The listing builds one solid part. Answer for the finished solid, in the listing's coordinates (mm). A direction names the side the tool comes from. Round coordinates to 2 decimals unless told otherwise and drop trailing zeros. Write each loop counter-clockwise with the first axis right and the second up, starting at its lowest first coordinate (ties: lowest second). Pieces come first, ordered by that corner, then holes.
(1) A cutting plane is placed at A-A, the plane y = -1. Give the vertices of the cut face in (x, z).
(2) A cutting plane is placed at B-B, the plane x = 16. Give the vertices of the cut face in (y, z), and give its area (3 significant figures).
(3) Find the intervals of material crossed by probe 1 along Z at (x, y) = (0, 12); probe 2 along Z at (x, y) = (6, -12); probe 3 along Z at (x, y) = (-20.5, -36), in increasing order.
(4) For faces 4 (the face through (-2.219, -15.021, 12.743)), 5 (the face through (20, -39.5, 10)), 6 (the face through (-16.8, -21, 11)), 7 (the face through (-12.897, -3.491, 19.947)), determine the directions among +Z, -Z, +X, -X, +Y, -Y from which every point of the face is accessible in a straight line to the end or side of a thin tool.
(5) A cutting plane is placed at D-D, the plane y = 5.5. Give the vertices of the cut face in (x, z).
(6) The mould has two halves that part along Y. Classify faces 1 (the face through (2.053, -3.491, 34.639)), 2 (the face through (1.3, -13.5, 12.9)), 3 (the face through (-22, -12, 22)): +Y half, -Y half, draft (parallel to the pull), parting line (faces both ways), or undercut.
(7) A cutting plane is placed at C-C, the plane y = -24.5. Give the number of separate pieces and of enclosed holes in the cut face, and give its area (3 significant figures).
from build123d import *

# Parameters (mm, degrees)
F0_R      = 2.05
F1_DEPTH  = 44
F2_R      = 4
F3_DEPTH  = 12.001
F4_DEPTH  = 6.8
F6_DEPTH  = 33.001
F7_R      = 2.05
F8_DEPTH  = 44.001
F9_DEPTH  = 8
F10_R     = 2
F11_DEPTH = 44.001
F12_DEPTH = 3.4
F13_R     = 3.6
F14_DEPTH = 4.2
F16_DEPTH = 44.001
F18_DEPTH = 44.001
F19_R     = 1.55
F20_DEPTH = 33.001
F21_DEPTH = 3


with BuildPart() as f1:
    # F0 (on Top) → F1 (new body)
    with BuildSketch(Plane.XY):
        Polygon((16.5, 16.5), (-16.5, 16.5), (-22, 16.5), (-22, -32.5), (-10, -32.5), (-10, -16.5), (8, -16.5), (8, -32.5), (22, -32.5), (22, 16.5), align=None)
        with Locations((-12, -12)):
            Circle(F0_R, mode=Mode.SUBTRACT)
        with Locations((12, -12)):
            Circle(F0_R, mode=Mode.SUBTRACT)
        with Locations((-12, 12)):
            Circle(F0_R, mode=Mode.SUBTRACT)
        with Locations((12, 12)):
            Circle(F0_R, mode=Mode.SUBTRACT)
    extrude(amount=F1_DEPTH)

    # F2 (on face) → F3 (cut, through all)
    with BuildSketch(Plane.YZ.offset(-10)):
        with Locations((-24.5, 36.4)):
            Circle(F2_R)
        with Locations((-24.5, 22)):
            Circle(F2_R)
        with Locations((-24.5, 7.6)):
            Circle(F2_R)
    extrude(amount=-F3_DEPTH, mode=Mode.SUBTRACT)

    # F2 (on face) → F4 (cut)
    with BuildSketch(Plane.YZ.offset(-10)):
        Polygon((-16.9944465005, 36.4), (-20.7472232503, 42.9), (-28.2527767497, 42.9), (-32.0055534995, 36.4), (-28.2527767497, 29.9), (-20.7472232503, 29.9), align=None)
        with Locations((-24.5, 36.4)):
            Circle(F2_R, mode=Mode.SUBTRACT)
        Polygon((-16.9944465005, 22), (-20.7472232503, 28.5), (-28.2527767497, 28.5), (-32.0055534995, 22), (-28.2527767497, 15.5), (-20.7472232503, 15.5), align=None)
        with Locations((-24.5, 22)):
            Circle(F2_R, mode=Mode.SUBTRACT)
        Polygon((-28.2527767497, 14.1), (-32.0055534995, 7.6), (-28.2527767497, 1.1), (-20.7472232503, 1.1), (-16.9944465005, 7.6), (-20.7472232503, 14.1), align=None)
        with Locations((-24.5, 7.6)):
            Circle(F2_R, mode=Mode.SUBTRACT)
    extrude(amount=-F4_DEPTH, mode=Mode.SUBTRACT)

    # F5 (on face) → F6 (cut, through all)
    with BuildSketch(Plane.XZ.offset(16.5)):
        Polygon((2.0710678119, 27), (-2.0710678119, 27), (-5, 24.0710678119), (-5, 19.9289321881), (-2.0710678119, 17), (2.0710678119, 17), (5, 19.9289321881), (5, 24.0710678119), align=None)
    extrude(amount=-F6_DEPTH, mode=Mode.SUBTRACT)

    # F7 (on face) → F8 (cut, through all)
    with BuildSketch(Plane(origin=(-22, 0, 0), x_dir=(0, -1, 0), z_dir=(-1, 0, 0))):
        with Locations((-12, 34)):
            Circle(F7_R)
        with Locations((12, 34)):
            Circle(F7_R)
        with Locations((12, 10)):
            Circle(F7_R)
        with Locations((-12, 10)):
            Circle(F7_R)
    extrude(amount=-F8_DEPTH, mode=Mode.SUBTRACT)

    # F9 (add): faces of the model
    f9_faces = [f1.faces().sort_by_distance(p)[0] for p in [
        (15, -32.5, 22),
        (-16, -32.5, 22),
    ]]
    extrude(f9_faces, amount=F9_DEPTH)

    # F10 (on face) → F11 (cut, through all)
    with BuildSketch(Plane.YZ.offset(22)):
        with Locations((-36, 10)):
            Circle(F10_R)
        with Locations((-36, 34)):
            Circle(F10_R)
    extrude(amount=-F11_DEPTH, mode=Mode.SUBTRACT)

    # F10 (on face) → F12 (cut)
    with BuildSketch(Plane.YZ.offset(22)):
        Polygon((-32.5, 7.9792740578), (-32.5, 12.0207259422), (-36, 14.0414518843), (-39.5, 12.0207259422), (-39.5, 7.9792740578), (-36, 5.9585481157), align=None)
        with Locations((-36, 10)):
            Circle(F10_R, mode=Mode.SUBTRACT)
        Polygon((-32.5, 31.9792740578), (-32.5, 36.0207259422), (-36, 38.0414518843), (-39.5, 36.0207259422), (-39.5, 31.9792740578), (-36, 29.9585481157), align=None)
        with Locations((-36, 34)):
            Circle(F10_R, mode=Mode.SUBTRACT)
    extrude(amount=-F12_DEPTH, mode=Mode.SUBTRACT)

    # F13 (on face) → F14 (cut)
    with BuildSketch(Plane(origin=(-22, 0, 0), x_dir=(0, -1, 0), z_dir=(-1, 0, 0))):
        with Locations((36, 10)):
            Circle(F13_R)
        with Locations((36, 34)):
            Circle(F13_R)
    extrude(amount=-F14_DEPTH, mode=Mode.SUBTRACT)

    # F15 (on face) → F16 (cut, through all)
    with BuildSketch(Plane(origin=(0, 0, 0), x_dir=(1, 0, 0), z_dir=(0, 0, -1))):
        Polygon((-4.05, -2.3382685902), (0, -4.6765371804), (4.05, -2.3382685902), (4.05, 2.3382685902), (0, 4.6765371804), (-4.05, 2.3382685902), align=None)
    extrude(amount=-F16_DEPTH, mode=Mode.SUBTRACT)

    # F17 (on face) → F18 (cut, through all)
    with BuildSketch(Plane(origin=(-22, 0, 0), x_dir=(0, -1, 0), z_dir=(-1, 0, 0))):
        Polygon((-2.3382685902, 17.95), (2.3382685902, 17.95), (4.6765371804, 22), (2.3382685902, 26.05), (-2.3382685902, 26.05), (-4.6765371804, 22), align=None)
    extrude(amount=-F18_DEPTH, mode=Mode.SUBTRACT)

    # F19 (on face) → F20 (cut, through all)
    with BuildSketch(Plane.XZ.offset(16.5)):
        with Locations((0, 30)):
            Circle(F19_R)
        with Locations((0, 14)):
            Circle(F19_R)
    extrude(amount=-F20_DEPTH, mode=Mode.SUBTRACT)

    # F19 (on face) → F21 (cut)
    with BuildSketch(Plane.XZ.offset(16.5)):
        Polygon((2.9444863729, 30), (1.4722431864, 32.55), (-1.4722431864, 32.55), (-2.9444863729, 30), (-1.4722431864, 27.45), (1.4722431864, 27.45), align=None)
        with Locations((0, 30)):
            Circle(F19_R, mode=Mode.SUBTRACT)
        Polygon((-1.4722431864, 16.55), (-2.9444863729, 14), (-1.4722431864, 11.45), (1.4722431864, 11.45), (2.9444863729, 14), (1.4722431864, 16.55), align=None)
        with Locations((0, 14)):
            Circle(F19_R, mode=Mode.SUBTRACT)
    extrude(amount=-F21_DEPTH, mode=Mode.SUBTRACT)


solid = f1.part
Solutions:
1. outline: (-22, 0) - (-4.05, 0) - (-4.05, 17.95) - (-22, 17.95) - close; (-22, 26.05) - (-4.05, 26.05) - (-4.05, 44) - (-22, 44) - close; (4.05, 0) - (22, 0) - (22, 17.95) - (4.05, 17.95) - close; (4.05, 26.05) - (22, 26.05) - (22, 44) - (4.05, 44) - close
2. outline: (-40.5, 0) - (16.5, 0) - (16.5, 44) - (-40.5, 44) - close; hole circle Ø4 at (-36, 10); hole circle Ø4 at (-36, 34); hole circle Ø4.1 at (-12, 10); hole circle Ø4.1 at (-12, 34); hole (-4.68, 22) - (-2.34, 17.95) - (2.34, 17.95) - (4.68, 22) - (2.34, 26.05) - (-2.34, 26.05) - close; hole circle Ø4.1 at (12, 10); hole circle Ø4.1 at (12, 34)
2. area: 2,370 mm2
3. probe 1: z = 0 to 7.95, 12.05 to 12.45, 15.55 to 17, 27 to 28.45, 31.55 to 31.95, 36.05 to 44
3. probe 2: z = 0 to 7.95, 12.05 to 31.95, 36.05 to 44
3. probe 3: z = 0 to 6.4, 13.6 to 30.4, 37.6 to 44
4. face 4: -Y
4. face 5: +X
4. face 6: none
4. face 7: +X, -X
5. outline: (-22, 0) - (22, 0) - (22, 44) - (-22, 44) - close; hole (-5, 19.93) - (-2.07, 17) - (2.07, 17) - (5, 19.93) - (5, 24.07) - (2.07, 27) - (-2.07, 27) - (-5, 24.07) - close; hole circle Ø3.1 at (0, 14); hole circle Ø3.1 at (0, 30)
6. face 1: undercut
6. face 2: -Y half
6. face 3: draft
7. separate pieces: 5
7. enclosed holes: 0
7. area: 754 mm2
